Part model, mm, in its own coordinate system. A direction names the side the tool comes from. Give positions to 0.01 mm unless a question says otherwise; leave off trailing zeros. Use one line per item in the form item = value. Start each with the question number.
1. Band-saw the part on A-A, the plane x = 7. State how many separate pieces and enclosed holes the cut face has, plus the area to 3 significant figures.
2. Drill centre lines: line 1 (Y direction, x = 6, z = -112.5); line 2 (Z direction, x = 10.5, y = 67.5); line 3 (Z direction, x = 4.25, y = 7.5). Where is each one in solid material? Low to high.
3. Pull direction Y, two halves, no side cores. Call faces 1 (the face through (5, 100, -76)), 2 (the face through (7.395, 94.186, -76.425)), 3 (the face through (5, 49, -155)): +Y half, -Y half, draft (parallel to the pull), parting line (faces both ways), or undercut.
4. Tool access for faces 4 (the face through (13.57, 14, 26.3)), 5 (the face through (7.395, 94.483, -42.76)), 6 (the face through (5, 12.5, 26)): list every direction of +Z, -Z, +X, -X, +Y, -Y with a clear straight run to the whole face (end or side of a thin tool).
5. Pin check, flat tips, straight feed: P1, Ø5, axis at y = 7.5, z = -147.5, coming from the +X side; P2, Ø6, axis at x = 2.5, z = 19, coming from the +Y side; P3, Ø4, axis at x = 4.5, z = 28, coming from the -Y side; P4, Ø4, axis at x = 11.5, y = 83, coming from the +Z side. Stop position of each tip, or through.
from build123d import *

# Parameters (mm, degrees)
SKETCH1_W           = 155
SKETCH1_H           = 100
BOSS_EXTRUDE1_DEPTH = 15
SKETCH2_W           = 15
SKETCH2_H           = 75
BOSS_EXTRUDE2_DEPTH = 75
SKETCH3_R           = 26
CUT_EXTRUDE1_DEPTH  = 75
CUT_EXTRUDE2_START  = -15
CUT_EXTRUDE2_DEPTH  = 15
FILLET1_R           = 15
SKETCH5_R           = 2
CUT_EXTRUDE3_DEPTH  = 186.067555233
FILLET7_R           = 5


# Read off the part's stored shape, not the designer's step: Cut-Extrude2
with BuildPart() as part:
    # Sketch1 → Boss-Extrude1 (new body)
    with BuildSketch(Plane(origin=(0, 0, 0), x_dir=(0, 0, -1), z_dir=(1, 0, 0))):
        with Locations((77.5, 50)):
            Rectangle(SKETCH1_W, SKETCH1_H)
    extrude(amount=BOSS_EXTRUDE1_DEPTH)

    # Sketch2 → Boss-Extrude2 (add)
    with BuildSketch(Plane.XY):
        with Locations((7.5, 50)):
            Rectangle(SKETCH2_W, SKETCH2_H)
    extrude(amount=BOSS_EXTRUDE2_DEPTH)

    # Sketch3 → Cut-Extrude1 (cut)
    with BuildSketch(Plane(origin=(15, 0, 0), x_dir=(0, 0, -1), z_dir=(1, 0, 0))):
        with Locations((-37.5, 50)):
            Circle(SKETCH3_R)
    extrude(amount=-CUT_EXTRUDE1_DEPTH, mode=Mode.SUBTRACT)

    # Cut-Extrude2 outline → Cut-Extrude2 (cut)
    with BuildSketch(Plane(origin=(15, 0, 0), x_dir=(0, 0, -1), z_dir=(1, 0, 0)).offset(CUT_EXTRUDE2_START)):
        with BuildLine():
            Line((-75, 12.5), (-37.5, 12.5))
            ThreePointArc((-37.5, 12.5), (-64.016504294, 23.483495706), (-75, 50))
            Line((-75, 50), (-75, 12.5))
        make_face()
        with BuildLine():
            Line((-75, 87.5), (-75, 50))
            ThreePointArc((-75, 50), (-64.016504294, 76.516504294), (-37.5, 87.5))
            Line((-37.5, 87.5), (-75, 87.5))
        make_face()
    extrude(amount=CUT_EXTRUDE2_DEPTH, mode=Mode.SUBTRACT)

    # Fillet1
    # the kernel refuses this fillet: 15 mm, written as the material it adds along each edge
    with BuildSketch(Plane(origin=(15, 12.5, 0), x_dir=(0, -1, 0), z_dir=(-1, 0, 0))) as fillet1_piece_1:
        with BuildLine():
            CenterArc((15, 14.790199458), FILLET1_R, 180, 80.405931773)
            Line((0, 14.790199458), (-0.3, 14.790199458))
            Line((-0.3, 14.790199458), (-0.3, 0))
            Line((-0.3, 0), (0, -0.3))
            ThreePointArc((0, -0.3), (6.25, -0.3), (12.45, -0.295803989))
            Line((12.45, -0.295803989), (12.5, 0))
        make_face()
    extrude(amount=15)
    with BuildSketch(Plane(origin=(0, 87.5, 0), x_dir=(0, 0, 1), z_dir=(1, 0, 0))) as fillet1_piece_2:
        with BuildLine():
            CenterArc((14.790199458, -15), FILLET1_R, 90, 80.405931773)
            Line((0, -12.5), (-0.295803989, -12.45))
            ThreePointArc((-0.295803989, -12.45), (-0.3, -6.25), (-0.3, 0))
            Line((-0.3, 0), (0, 0.3))
            Line((0, 0.3), (14.790199458, 0.3))
            Line((14.790199458, 0.3), (14.790199458, 0))
        make_face()
    extrude(amount=15)

    # Sketch5 → Cut-Extrude3 (cut, through all)
    with BuildSketch(Plane.ZY):
        with Locations((-147.5, 92.5)):
            Circle(SKETCH5_R)
        with Locations((-112.5, 92.5)):
            Circle(SKETCH5_R)
        with Locations((-77.5, 92.5)):
            Circle(SKETCH5_R)
        with Locations((-42.5, 92.5)):
            Circle(SKETCH5_R)
        with Locations((-7.5, 92.5)):
            Circle(SKETCH5_R)
        with Locations(Location((-7.5, 7.5, 0), (0, 0, 180))):
            Circle(SKETCH5_R)
        with Locations(Location((-42.5, 7.5, 0), (0, 0, 180))):
            Circle(SKETCH5_R)
        with Locations(Location((-77.5, 7.5, 0), (0, 0, 180))):
            Circle(SKETCH5_R)
        with Locations(Location((-112.5, 7.5, 0), (0, 0, 180))):
            Circle(SKETCH5_R)
        with Locations(Location((-147.5, 7.5, 0), (0, 0, 180))):
            Circle(SKETCH5_R)
        with Locations(Location((-147.5, 37.5, 0), (0, 0, 180))):
            Circle(SKETCH5_R)
        with Locations(Location((-147.5, 67.5, 0), (0, 0, 180))):
            Circle(SKETCH5_R)
    extrude(amount=-CUT_EXTRUDE3_DEPTH, mode=Mode.SUBTRACT)

    # Fillet7
    fillet7_edges = [part.edges().sort_by_distance(p)[0] for p in [
        (15, 50, -155),
        (15, 100, -77.5),
        (15, 12.5, 26.145099729),
        (15, 87.5, 26.145099729),
        (15, 76.516504294, 64.016504294),
        (15, 8.956439237, 5.107741092),
        (15, 91.043560763, 5.107741092),
        (15, 0, -77.5),
    ]]
    fillet(fillet7_edges, radius=FILLET7_R)


solid = part.part
From the geometry:
q1.separate_pieces = 1
q1.enclosed_holes = 13
q1.area = 18,300 mm²
q2.line_1 = 0 to 5.5, 9.5 to 90.5, 94.5 to 100
q2.line_2 = -154.97 to -149.5, -145.5 to 18.27, 56.73 to 70.64
q2.line_3 = -155 to -149.5, -145.5 to -114.5, -110.5 to -79.5, -75.5 to -44.5, -40.5 to -9.5, -5.5 to 3.61
q3.face_1 = +Y half
q3.face_2 = undercut
q3.face_3 = draft
q4.face_4 = +Z, +X, -Y
q4.face_5 = +X, -X
q4.face_6 = +Z, +X, -X, -Y
q5.P1 = 15
q5.P2 = 87.5
q5.P3 = 12.5
q5.P4 = 58.33
